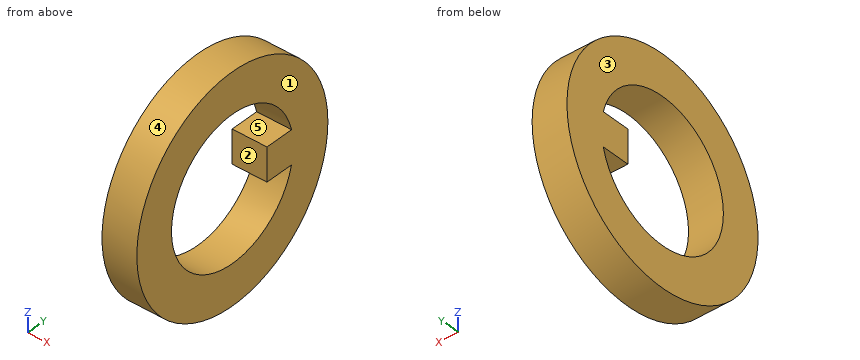
Autodesk Inventor part; units mm, degrees
ref_plane "YZ Plane" through (0, 0, 0) normal (1, 0, 0) x (0, 1, 0)
ref_plane "XZ Plane" through (0, 0, 0) normal (0, 1, 0) x (-1, 0, 0)
ref_plane "XY Plane" through (0, 0, 0) normal (0, 0, 1) x (1, 0, 0)
sketch "Sketch1" plane through (0, 0, 0) normal (1, 0, 0) x (0, 1, 0)
  circle A0 centre (0, 0) radius 6.477
  line L0 (9.271, 1.524) -> (9.271, -1.524)
  line L1 (9.271, -1.524) -> (3.683, -1.524)
  line L2 (3.683, -1.524) -> (3.683, 1.524)
  line L3 (3.683, 1.524) -> (9.271, 1.524)
  line L4 (9.271, 1.524) -> (3.683, -1.524) construction
  line L5 (9.271, -1.524) -> (3.683, 1.524) construction
  circle A1 centre (0, 0) radius 10.16
  line L6 (9.271, 1.524) -> (10.045, 1.524)
  line L7 (9.271, -1.524) -> (10.045, -1.524)
  point P0 (6.477, 0)
  point P1 (6.2952, -1.524)
  point P2 (6.2952, 1.524)
  dimension "d0" = 12.954
  dimension "d1" = 3.048
  dimension "d2" = 5.588
  dimension "d3" = 20.32
extrude "Extrusion1" add sketch "Sketch1" along normal blind 3.175 contours A0 L1 L2 L3 | A0 L3 L0 L1 | A0 L1 L7 A1 L6 L3 | L6 A1 L7 L0 picked at (4.6143, 0)
properties part number "handle insert cover"
Input: part model. Units: mm. Frame: model coordinates. Face numbers are marked on the shaded views. A direction names the side the tool comes from. Give positions to 0.01 mm unless a question says otherwise; leave off trailing zeros. Order: outer loops, then holes, each group sorted by start corner. A loop starts at its lowest first (then second) coordinate and runs counter-clockwise, first axis right, second up.
1. Section C-C on y = 6. Return the cut outline in (x, z) (3 decimals).
Derived:
outline: (0, -8.199) - (3.175, -8.199) - (3.175, -2.44) - (0, -2.44) - close; (0, -1.524) - (3.175, -1.524) - (3.175, 1.524) - (0, 1.524) - close; (0, 2.44) - (3.175, 2.44) - (3.175, 8.199) - (0, 8.199) - close
2. Mould query, pull axis Z, two halves, no side actions, for the marked faces 3, 4 and 5. Classes: released by +Z, released by -Z, zero draft, split by the parting line, or undercut.
Derived:
face 3: zero draft
face 4: split by the parting line
face 5: undercut
3. Section B-B on z = 0. Return the cut outline in (x, y) (3 decimals).
Derived:
outline: (0, -10.16) - (3.175, -10.16) - (3.175, -6.477) - (0, -6.477) - close; (0, 3.683) - (3.175, 3.683) - (3.175, 10.16) - (0, 10.16) - close
4. Pin query (flat end, axial travel): pin 1 (3 mm diameter, centred on y = -2, z = -4.5, fed in from -X); pin 2 (1.5 mm diameter, centred on x = 1.5, y = -8, fed in from -Z); pin 3 (1.3 mm diameter, centred on x = 1, y = 5, fed in from +Z); pin 4 (1 mm diameter, centred on x = 3, y = -4.5, fed in from +Z). Return the tip coordinate at first contact, or that it passes through.
Derived:
pin 1: passes through
pin 2: stops at z = -7.12
pin 3: stops at z = 9.18
pin 4: stops at z = 9.34
5. Reachability of the marked faces 1 and 2 from +Z, -Z, +X, -X, +Y, -Y: full face, straight path, thin tool, end or side. Return the list, or none.
Derived:
face 1: +Z, -Z, +X, +Y, -Y
face 2: +X, -X
6. Section A-A on y = 0. Return the cut outline in (x, z) (3 decimals), and give its area (3 significant figures).
Derived:
outline: (0, -10.16) - (3.175, -10.16) - (3.175, -6.477) - (0, -6.477) - close; (0, 6.477) - (3.175, 6.477) - (3.175, 10.16) - (0, 10.16) - close
area: 23.4 mm2
7. Material intervals for L1, parallel to Z at x = 0.7, y = 0; L2, parallel to Y at x = 2.4, z = 0; L3, parallel to Y at x = 3, z = 3.25, sorted ascending.
Derived:
L1: z = -10.16 to -6.48, 6.48 to 10.16
L2: y = -10.16 to -6.48, 3.68 to 10.16
L3: y = -9.63 to -5.6, 5.6 to 9.63
8. Section D-D on x = 2.4. Return the cut outline in (y, z), and give its area (3 significant figures).
Derived:
outline: circle Ø20.32 at (0, 0); hole (3.68, -1.52) - (3.68, 1.52) - (6.3, 1.52) arc R6.48 ccw (long way) to (6.3, -1.52) - close
area: 201 mm2
